from build123d import *

# Parameters (mm, degrees)
SKETCH1_R               = 1
BOSS_EXTRUDE1_DEPTH     = 10
SKETCH5_R               = 3.5
SKETCH5_R_2             = 2
BOSS_EXTRUDE3_DEPTH     = 8
CUT_EXTRUDE1_DEPTH      = 20.949878445
CUT_EXTRUDE1_DEPTH_BACK = 20.949878445
SKETCH6_R               = 1


with BuildPart() as part:
    # Sketch1 → Boss-Extrude1 (new body)
    with BuildSketch(Plane.XY):
        with BuildLine():
            Line((-1.390653283, 13.224086579), (-2, 8.261355821))
            ThreePointArc((-2, 8.261355821), (-2.767329313, -8.036907893), (6.66222002, 5.278714276))
            Line((6.66222002, 5.278714276), (9.237410395, 9.564550779))
            ThreePointArc((9.237410395, 9.564550779), (8.899037344, 11.390248383), (7.045710912, 11.276894083))
            Line((7.045710912, 11.276894083), (3.510177006, 7.741360177))
            ThreePointArc((3.510177006, 7.741360177), (2.767329313, 8.036907893), (2, 8.261355821))
            Line((2, 8.261355821), (1.390653283, 13.224086579))
            ThreePointArc((1.390653283, 13.224086579), (0, 14.454432673), (-1.390653283, 13.224086579))
        make_face()
        Circle(SKETCH1_R, mode=Mode.SUBTRACT)
    extrude(amount=BOSS_EXTRUDE1_DEPTH)

    # Sketch5 → Boss-Extrude3 (add)
    with BuildSketch(Plane(origin=(0, 0, 0), x_dir=(-1, 0, 0), z_dir=(0, 0, -1))):
        with Locations(Location((0, 0, 0), (0, 0, 180))):
            Circle(SKETCH5_R)
        Circle(SKETCH5_R_2, mode=Mode.SUBTRACT)
    extrude(amount=BOSS_EXTRUDE3_DEPTH)

    # Sketch6 → Cut-Extrude1 (cut, two sides: drawn at the far end of the back side and taken through both)
    with BuildSketch(Plane(origin=(0, 0, 0), x_dir=(0, 0, -1), z_dir=(1, 0, 0)).offset(-CUT_EXTRUDE1_DEPTH_BACK)):
        with Locations((2.5, 0)):
            Circle(SKETCH6_R)
    extrude(amount=CUT_EXTRUDE1_DEPTH + CUT_EXTRUDE1_DEPTH_BACK, mode=Mode.SUBTRACT)


solid = part.part
Source: CAD feature listing. Evaluate the final solid. Frame: model axes, mm. A direction names the side the tool comes from. Coordinates: 2 decimals unless noted, no trailing zeros. Order: outer loops, then holes, each group sorted by start corner. A loop starts at its lowest first (then second) coordinate and runs counter-clockwise, first axis right, second up. Notation, with made-up numbers: M -32.5,74 L -13.5,74 A22 ccw -13.5,113 Z; hole C 5.5,-34.5 d8. An arc over 180 degrees is marked long. Write each question's results on one line, items separated by ' | '. Start each with the question number.
1. Section B-B, the plane z = 8.5. Return the cut outline in (x, y).
2. Pin query (flat end, axial travel): pin 1 (3 mm diameter, centred on x = 0, y = 0, fed in from -Z); pin 2 (8 mm diameter, centred on x = 7, z = 6, fed in from +Y); pin 3 (2 mm diameter, centred on x = 3, z = -4, fed in from -Y); pin 4 (1.8 mm diameter, centred on y = 0, z = -2.5, fed in from -X). Return the tip coordinate at first contact, or that it passes through.
3. Section A-A, the plane x = 0. Return the cut outline in (y, z), then the cut area to 3 significant figures.
4. Section C-C, the plane y = 0. Return the cut outline in (x, z), then the cut area to 3 significant figures.
5. Reachability of faces 4 (the face through (2.6, 0.84, -3.04)), 5 (the face through (1, -1, 0)), 6 (the face through (8.921, 11.373, 4.93)), 7 (the face through (1.7, 10.7, 4.9)), 8 (the face through (7.93, 7.39, 4.93)) from +Z, -Z, +X, -X, +Y, -Y: full face, straight path, thin tool, end or side. Return the list, or none.
6. Draft query along X for faces 1 (the face through (2.3, 3.1, 0)), 2 (the face through (5.3, 9.53, 4.93)), 3 (the face through (3.34, -1.05, -3.94)). Return one class per face: +X half, -X half, draft (parallel to the pull), parting line (faces both ways), or undercut.
7. Material intervals for L1, parallel to Z at x = -2.95, y = 0; L2, parallel to Z at x = -0.5, y = -1.5; L3, parallel to Y at x = -2.85, z = -2.5, sorted ascending.
8. Section D-D, the plane z = -2.5. Return the cut outline in (x, y).
Solution:
1) outline: M -2,8.26 A8.5 ccw long 6.66,5.28 L 9.24,9.56 A1.4 ccw 7.05,11.28 L 3.51,7.74 A8.5 ccw 2,8.26 L 1.39,13.22 A1.4 ccw -1.39,13.22 Z; hole C 0,0 d2
2) pin 1: z = 0 | pin 2: y = 11.69 | pin 3: y = -2.87 | pin 4: through
3) outline: M -8.5,0 L -3.5,0 L -3.5,-8 L -2,-8 L -2,0 L -1,0 L -1,10 L -8.5,10 Z; M 1,0 L 2,0 L 2,-8 L 3.5,-8 L 3.5,0 L 14.45,0 L 14.45,10 L 1,10 Z | area: 234 mm²
4) outline: M -8.5,0 L -3.5,0 L -3.5,-1.5 L -2,-1.5 L -2,0 L -1,0 L -1,10 L -8.5,10 Z; M -3.5,-8 L -2,-8 L -2,-3.5 L -3.5,-3.5 Z; M 1,0 L 2,0 L 2,-1.5 L 3.5,-1.5 L 3.5,0 L 8.5,0 L 8.5,10 L 1,10 Z; M 2,-8 L 3.5,-8 L 3.5,-3.5 L 2,-3.5 Z | area: 168 mm²
5) face 4: +X, -X | face 5: -Z | face 6: +Z, -Z | face 7: +Z, -Z, +Y | face 8: +Z, -Z, +X
6) face 1: draft | face 2: undercut | face 3: parting line
7) L1: -8 to -3.5, -1.5 to 10 | L2: 0 to 10 | L3: -2.03 to -1, 1 to 2.03
8) outline: M -3.35,-1 A3.5 ccw 3.35,-1 L 1.73,-1 A2 cw -1.73,-1 Z; M -3.35,1 L -1.73,1 A2 cw 1.73,1 L 3.35,1 A3.5 ccw Z
